Geometry check sheet. Reference: the model listing, model coordinates, mm. Face numbers are marked on the shaded views. A direction names the side the tool comes from. Coordinates: 2 decimals unless noted, no trailing zeros. Write each loop counter-clockwise with the first axis right and the second up, starting at its lowest first coordinate (ties: lowest second). Pieces come first, ordered by that corner, then holes.
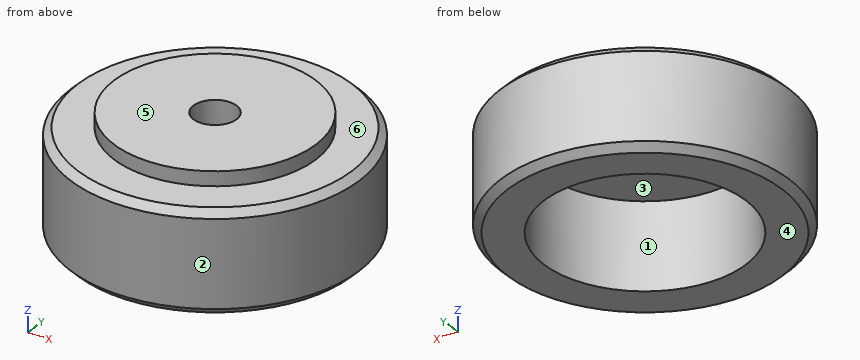
from build123d import *

# Parameters (mm, degrees)
F0_R     = 7
F1_DEPTH = 1
F0_R_2   = 10
F2_DEPTH = 7
F3_SIZE  = 0.5
F4_R     = 7
F4_R_2   = 1.5
F5_DEPTH = 6
F6_DEPTH = 25


with BuildPart() as f1:
    # F0 (on Top) → F1 (new body)
    with BuildSketch(Plane.XY):
        Circle(F0_R)
    extrude(amount=F1_DEPTH)

    # F0 (on Top) → F2 (join)
    with BuildSketch(Plane.XY):
        Circle(F0_R_2)
        Circle(F0_R, mode=Mode.SUBTRACT)
        Circle(F0_R)
    extrude(amount=-F2_DEPTH)

    # F3
    f3_edges = [f1.edges().sort_by_distance(p)[0] for p in [
        (-10, 0, 0),
        (-10, 0, -7),
    ]]
    chamfer(f3_edges, length=F3_SIZE)

    # F4 (on face) → F5 (cut)
    with BuildSketch(Plane(origin=(0, 0, -7), x_dir=(1, 0, 0), z_dir=(0, 0, -1))):
        Circle(F4_R)
        Circle(F4_R_2, mode=Mode.SUBTRACT)
        Circle(F4_R_2)
    extrude(amount=-F5_DEPTH, mode=Mode.SUBTRACT)

    # F4 (on face) → F6 (cut)
    with BuildSketch(Plane(origin=(0, 0, -7), x_dir=(1, 0, 0), z_dir=(0, 0, -1))):
        Circle(F4_R_2)
    extrude(amount=-F6_DEPTH, mode=Mode.SUBTRACT)


solid = f1.part
1. Gauge pin test, flat ends, axial feed: pin 1 Ø1 at (y, z) = (5.5, -0.5) entering from +X; pin 2 Ø2 at (x, z) = (-6.5, 0) entering from -Y; pin 3 Ø1.5 at (y, z) = (-0.5, 0) entering from +X; pin 4 Ø4 at (x, z) = (-7.5, -2.5) entering from -Y. Record the tip position at first contact, or that the pin passes through.
Computed values:
pin 1: stops at x = 8.66
pin 2: stops at y = -8.26
pin 3: stops at x = 10
pin 4: stops at y = -8.35
2. Sectioned sample at B-B, the plane z = -5.25. Record the boundary of the cut face in (x, y), and give its area (3 significant figures).
Computed values:
outline: circle Ø20 at (0, 0); hole circle Ø14 at (0, 0)
area: 160 mm2
3. Thickness scan on line 1 along Y through (x, z) = (0, -4.75); line 2 along Z through (x, y) = (0.75, 7.5). Record the ranges inside material, lowest first.
Computed values:
line 1: y = -10 to -7, 7 to 10
line 2: z = -7 to 0
4. Access from +Z, -Z, +X, -X, +Y, -Y to the whole of each face (thin tool, end or side, straight path). Record for the marked faces 5 and 6.
Computed values:
face 5: +Z, +X, -X, +Y, -Y
face 6: +Z
5. Draft check along Y on the marked faces 1, 2, 3 and 4. Enter one of: released by +Y, released by -Y, zero draft, split by the parting line, or undercut.
Computed values:
face 1: undercut
face 2: split by the parting line
face 3: undercut
face 4: zero draft
6. Sectioned sample at A-A, the plane x = 0. Record the boundary of the cut face in (y, z).
Computed values:
outline: (-10, -6.5) - (-9.5, -7) - (-7, -7) - (-7, -1) - (-1.5, -1) - (-1.5, 1) - (-7, 1) - (-7, 0) - (-9.5, 0) - (-10, -0.5) - close; (1.5, -1) - (7, -1) - (7, -7) - (9.5, -7) - (10, -6.5) - (10, -0.5) - (9.5, 0) - (7, 0) - (7, 1) - (1.5, 1) - close
